from build123d import *

# Parameters (mm, degrees)
SKETCH2_W           = 35
SKETCH2_H           = 20
SKETCH2_R           = 1.5
BOSS_EXTRUDE1_DEPTH = 5
SKETCH3_R           = 3
CUT_EXTRUDE1_DEPTH  = 3


with BuildPart() as part:
    # Sketch2 → Boss-Extrude1 (new body)
    with BuildSketch(Plane(origin=(0, 0, 0), x_dir=(1, 0, 0), z_dir=(0, 1, 0))):
        Rectangle(SKETCH2_W, SKETCH2_H)
        with Locations(Location((-13.05, 0, 0), (0, 0, 270))):
            Circle(SKETCH2_R, mode=Mode.SUBTRACT)
        with Locations(Location((13.05, 0, 0), (0, 0, 270))):
            Circle(SKETCH2_R, mode=Mode.SUBTRACT)
    extrude(amount=BOSS_EXTRUDE1_DEPTH)

    # Sketch3 → Cut-Extrude1 (cut)
    with BuildSketch(Plane(origin=(0, 5, 0), x_dir=(1, 0, 0), z_dir=(0, 1, 0))):
        with Locations(Location((-13.05, 0, 0), (0, 0, 270))):
            Circle(SKETCH3_R)
        with Locations(Location((13.05, 0, 0), (0, 0, 270))):
            Circle(SKETCH3_R)
    extrude(amount=-CUT_EXTRUDE1_DEPTH, mode=Mode.SUBTRACT)


solid = part.part
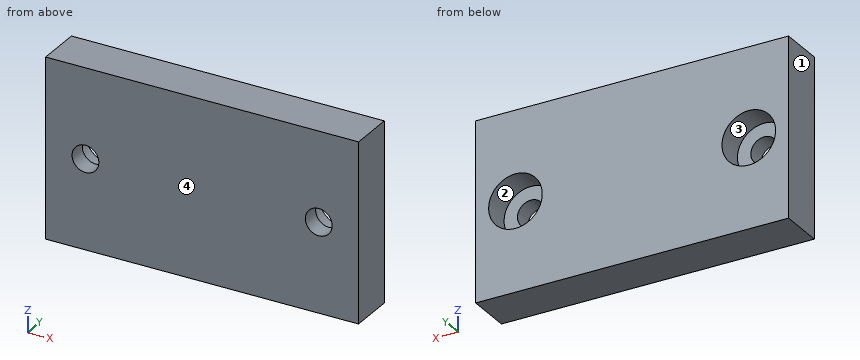
Could you check a few things on this model? Use its own coordinates, in mm. Face numbers are marked on the shaded views. Give positions to 0.01 mm unless a question says otherwise; leave off trailing zeros. Order: outer loops, then holes, each group sorted by start corner. A loop starts at its lowest first (then second) coordinate and runs counter-clockwise, first axis right, second up.
1. Suppose I cut it at A-A (z = 0). List the corners of the cut face in (x, y) for me.
2. Suppose I cut it at B-B (x = -13.05). List the corners of the cut face in (y, z) for me, plus the area to 3 significant figures.
3. I need wall thicknesses on L1, parallel to X at y = 3.4, z = 0; L2, parallel to X at y = 1, z = 0; L3, parallel to Z at x = 13, y = 3.8. Which ranges of each line are inside material? Lowest first, please.
4. Suppose I cut it at D-D (y = 1.55). List the corners of the cut face in (x, z) for me, plus the area to 3 significant figures.
5. We'd pull the mould along X, two halves only. Please class the marked faces 1, 2, 3 and 4: pulls with the +X half, pulls with the -X half, needs draft (parallel to the pull), parting line crosses it, or undercut.
6. Suppose I cut it at C-C (y = 4.5). List the corners of the cut face in (x, z) for me.
Solved:
1. outline: (-17.5, 0) - (-14.55, 0) - (-14.55, 2) - (-16.05, 2) - (-16.05, 5) - (-17.5, 5) - close; (-11.55, 0) - (11.55, 0) - (11.55, 2) - (10.05, 2) - (10.05, 5) - (-10.05, 5) - (-10.05, 2) - (-11.55, 2) - close; (14.55, 0) - (17.5, 0) - (17.5, 5) - (16.05, 5) - (16.05, 2) - (14.55, 2) - close
2. outline: (0, -10) - (5, -10) - (5, -3) - (2, -3) - (2, -1.5) - (0, -1.5) - close; (0, 1.5) - (2, 1.5) - (2, 3) - (5, 3) - (5, 10) - (0, 10) - close
2. area: 76.0 mm2
3. L1: x = -17.5 to -16.05, -10.05 to 10.05, 16.05 to 17.5
3. L2: x = -17.5 to -14.55, -11.55 to 11.55, 14.55 to 17.5
3. L3: z = -10 to -3, 3 to 10
4. outline: (-17.5, -10) - (17.5, -10) - (17.5, 10) - (-17.5, 10) - close; hole circle Ø3 at (-13.05, 0); hole circle Ø3 at (13.05, 0)
4. area: 686 mm2
5. face 1: pulls with the -X half
5. face 2: undercut
5. face 3: undercut
5. face 4: needs draft
6. outline: (-17.5, -10) - (17.5, -10) - (17.5, 10) - (-17.5, 10) - close; hole circle Ø6 at (-13.05, 0); hole circle Ø6 at (13.05, 0)
